from build123d import *

# Parameters (mm, degrees)
F0_W     = 800.1
F0_H     = 76.2
F0_R     = 12.7
F1_DEPTH = 5.08
F2_W     = 800.1
F2_H     = 5.08
F3_DEPTH = 19.05


with BuildPart() as f1:
    # F0 (on Front) → F1 (new body)
    with BuildSketch(Plane.XZ):
        with Locations((7.7429, -39.377729)):
            Rectangle(F0_W, F0_H)
        with Locations((255.3929, -39.377729)):
            Circle(F0_R, mode=Mode.SUBTRACT)
        with Locations((-239.9071, -39.377729)):
            Circle(F0_R, mode=Mode.SUBTRACT)
    extrude(amount=F1_DEPTH)

    # F2 (on face) → F3 (join)
    with BuildSketch(Plane.XZ.offset(5.08)):
        with Locations((7.7429, -3.817729)):
            Rectangle(F2_W, F2_H)
    extrude(amount=F3_DEPTH)


solid = f1.part
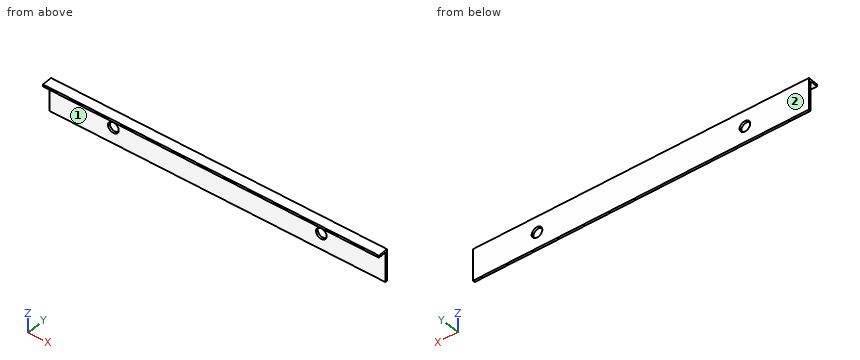
Can you work these out from the model? Positions are in its coordinate system, mm. Face numbers are marked on the shaded views. A direction names the side the tool comes from. Give positions to 0.01 mm unless a question says otherwise; leave off trailing zeros. Order: outer loops, then holes, each group sorted by start corner. A loop starts at its lowest first (then second) coordinate and runs counter-clockwise, first axis right, second up. Notation, with made-up numbers: M 67,52.5 L 105,52.5 A10 ccw 105,64.5 Z; hole C 62,15 d6. An arc over 180 degrees is marked long. Use a Markdown table: item, result. Add a question column.
Item 1: Will these pins go through, and if not, where does the flat tip stop? pin 1 (3 mm diameter, centred on x = -7, z = -43.5, fed in from -Y); pin 2 (6 mm diameter, centred on y = -10.5, z = -50, fed in from -X); pin 3 (9.5 mm diameter, centred on x = 2, y = -16, fed in from -Z).
Item 2: Suppose I cut it at A-A (x = 260). List the corners of the cut face in (y, z) for me, then the cut area to 3 significant figures.
Item 3: Suppose I cut it at C-C (z = -20). List the corners of the cut face in (x, y) for me, then the cut area to 3 significant figures.
Item 4: For the marked faces 1 and 2, which set-ups out of +Z, -Z, +X, -X, +Y, -Y let a thin tool reach every point of the face, with its end or its side?
Item 5: Suppose I cut it at B-B (x = 149.5). List the corners of the cut face in (y, z) for me, then the cut area to 3 significant figures.
Item 6: If I drill on L1, parallel to X at y = -5, z = -47.5; L2, parallel to Z at x = 37.5, y = -13.5; L3, parallel to Y at x = -296, z = -9, over which ranges is the centre line in solid material (lowest first)? Write a range as [from, to].
Item 7: Suppose I cut it at D-D (y = -17). List the corners of the cut face in (x, z) for me, then the cut area to 3 significant figures.
Answer sheet:
| question | item | result |
|---|---|---|
| 1 | pin 1 | stops at y = -5.08 |
| 1 | pin 2 | passes through |
| 1 | pin 3 | stops at z = -6.36 |
| 2 | outline | M -24.13,-6.36 L -5.08,-6.36 L -5.08,-27.54 L 0,-27.54 L 0,-1.28 L -24.13,-1.28 Z; M -5.08,-77.48 L 0,-77.48 L 0,-51.21 L -5.08,-51.21 Z |
| 2 | area | 364 mm² |
| 3 | outline | M -392.31,-5.08 L 407.79,-5.08 L 407.79,0 L -392.31,0 Z |
| 3 | area | 4,060 mm² |
| 4 | face 1 | -Z, +X, -X, -Y |
| 4 | face 2 | +Z, -Z, +X, -X, +Y |
| 5 | outline | M -24.13,-6.36 L -5.08,-6.36 L -5.08,-77.48 L 0,-77.48 L 0,-1.28 L -24.13,-1.28 Z |
| 5 | area | 484 mm² |
| 6 | L1 | x = [-392.31, -249.67], [-230.14, 245.63], [265.16, 407.79] |
| 6 | L2 | z = [-6.36, -1.28] |
| 6 | L3 | y = [-5.08, 0] |
| 7 | outline | M -392.31,-6.36 L 407.79,-6.36 L 407.79,-1.28 L -392.31,-1.28 Z |
| 7 | area | 4,060 mm² |
